```python
from build123d import *

# Parameters (mm, degrees)
F0_W      = 152.4
F0_H      = 152.4
F0_W_2    = 147.32
F0_H_2    = 147.32
F1_DEPTH  = 101.6
F2_W      = 152.4
F2_H      = 152.4
F3_DEPTH  = 2.54
F4_W      = 27.94
F4_H      = 18.1844604351
F4_H_2    = 17.9737907264
F5_DEPTH  = 25.4
F7_DEPTH  = 101.6
F8_W      = 25.4
F8_H      = 5.08
F9_DEPTH  = 101.6
F10_W     = 25.4
F10_H     = 5.08
F11_DEPTH = 101.6
F12_W     = 5.08
F12_H     = 5.08
F13_DEPTH = 101.6
F14_W     = 38.1
F14_H     = 5.08
F15_DEPTH = 101.6
F16_W     = 5.08
F16_H     = 38.4063468442
F16_H_2   = 5.08
F17_DEPTH = 101.6
F18_W     = 25.4
F18_H     = 104.14
F19_DEPTH = 25.4
F20_R     = 5.07999
F21_W     = 5.08
F21_H     = 5.08
F21_W_2   = 38.1
F21_H_2   = 22.86
F22_DEPTH = 101.6
F23_R     = 1.016
F24_DEPTH = 15.24


# Not quite as in the source:
# - a fillet or chamfer is up to 0.001 mm smaller than in the source, because OpenCascade refuses the exact size


with BuildPart() as f1:
    # F0 (on Top) → F1 (new body)
    with BuildSketch(Plane.XY):
        with Locations((-4.47035e-05, 5.21541e-05)):
            Rectangle(F0_W, F0_H)
        with Locations((-4.47035e-05, 5.21541e-05)):
            Rectangle(F0_W_2, F0_H_2, mode=Mode.SUBTRACT)
    extrude(amount=F1_DEPTH)

    # F2 (on face) → F3 (join)
    with BuildSketch(Plane(origin=(0, 0, 0), x_dir=(1, 0, 0), z_dir=(0, 0, -1))):
        with Locations((-4.47035e-05, -5.21541e-05)):
            Rectangle(F2_W, F2_H)
    extrude(amount=F3_DEPTH)

    # F4 (on face) → F5 (cut)
    with BuildSketch(Plane.XZ.offset(76.1999478459)):
        with Locations((44.4499552965, 25.6276302175)):
            Rectangle(F4_W, F4_H)
        with Locations((-44.4500447035, 25.5222953632)):
            Rectangle(F4_W, F4_H_2)
    extrude(amount=-F5_DEPTH, mode=Mode.SUBTRACT)

    # F6 (on face) → F7 (join)
    with BuildSketch(Plane.XY):
        Polygon((-17.7800447035, 58.4200521541), (-17.7800447035, -50.7999478459), (-12.7000447035, -50.7999478459), (-12.7000447035, 53.3400521541), (12.6999552965, 53.3400521541), (12.6999552965, -50.7999478459), (17.7799552965, -50.7999478459), (17.7799552965, 44.5264838636), (17.7799552965, 58.4200521541), align=None)
    extrude(amount=F7_DEPTH)

    # F8 (on face) → F9 (join)
    with BuildSketch(Plane.XY):
        with Locations((-4.47035e-05, -48.2599478459)):
            Rectangle(F8_W, F8_H)
    extrude(amount=F9_DEPTH)

    # F10 (on face) → F11 (cut)
    with BuildSketch(Plane.XY.offset(101.6)):
        with Locations((-4.47035e-05, 55.8800521541)):
            Rectangle(F10_W, F10_H)
    extrude(amount=-F11_DEPTH, mode=Mode.SUBTRACT)

    # F12 (on face) → F13 (join)
    with BuildSketch(Plane.XY):
        with Locations((-20.3200447035, 14.9337053099)):
            Rectangle(F12_W, F12_H)
    extrude(amount=F13_DEPTH)

    # F14 (on face) → F15 (join)
    with BuildSketch(Plane.XY):
        with Locations((-54.6100447035, 14.9337053099)):
            Rectangle(F14_W, F14_H)
    extrude(amount=F15_DEPTH)

    # F16 (on face) → F17 (join)
    with BuildSketch(Plane.XY):
        with Locations((-43.1800447035, 36.676878732)):
            Rectangle(F16_W, F16_H)
        with Locations((-43.1800447035, 71.1200521541)):
            Rectangle(F16_W, F16_H_2)
        with Locations((43.1799552965, 71.1200521541)):
            Rectangle(F16_W, F16_H_2)
        with Locations((43.1799552965, 36.676878732)):
            Rectangle(F16_W, F16_H)
    extrude(amount=F17_DEPTH)

    # F18 (on face) → F19 (cut)
    with BuildSketch(Plane.XY):
        with Locations((-4.47035e-05, 6.3500521541)):
            Rectangle(F18_W, F18_H)
    extrude(amount=-F19_DEPTH, mode=Mode.SUBTRACT)

    # F20 (radius 5.08 in the source; OpenCascade refuses exactly that, so slightly less here)
    f20_edges = [f1.edges().sort_by_distance(p)[0] for p in [
        (-17.780045, 58.420052, 50.8),
        (17.779955, 58.420052, 50.8),
    ]]
    fillet(f20_edges, radius=F20_R)

    # F21 (on face) → F22 (join)
    with BuildSketch(Plane.XY):
        with Locations((20.3199552965, 14.9337053099)):
            Rectangle(F21_W, F21_H)
        with Locations((54.6099552965, 14.9337053099)):
            Rectangle(F21_W_2, F21_H)
        with Locations((-15.2400447035, -62.2299478459)):
            Rectangle(F21_W, F21_H_2)
        with Locations((15.2399552965, -71.1199478459)):
            Rectangle(F21_W, F21_H)
    extrude(amount=F22_DEPTH)

    # F23 (on face) → F24 (cut)
    with BuildSketch(Plane(origin=(0, 0, -2.54), x_dir=(1, 0, 0), z_dir=(0, 0, -1))):
        with Locations((-74.9300447035, 74.9299478459)):
            Circle(F23_R)
        with Locations((74.9299552965, 74.9299478459)):
            Circle(F23_R)
        with Locations((-74.9300447035, -74.9300521541)):
            Circle(F23_R)
        with Locations((74.9299552965, -74.9300521541)):
            Circle(F23_R)
    extrude(amount=-F24_DEPTH, mode=Mode.SUBTRACT)


solid = f1.part
```
Build history of the part. All positions in model axes, mm. A direction names the side the tool comes from. Round coordinates to 2 decimals unless told otherwise and drop trailing zeros. Write each loop counter-clockwise with the first axis right and the second up, starting at its lowest first coordinate (ties: lowest second). Pieces come first, ordered by that corner, then holes.
1) Band-saw the part on A-A, the plane x = -9. List the corners of the cut face in (y, z), and give its area (3 significant figures).
2) Band-saw the part on B-B, the plane y = 41.5. List the corners of the cut face in (x, z), and give its area (3 significant figures).
3) Drill centre lines: probe 1 along X at (y, z) = (70, 89.5); probe 2 along Y at (x, z) = (7, 63.5); probe 3 along X at (y, z) = (31, 22). Where is each one in solid material? Low to high.
4) Mould opens along Y. For faces 3 (the flat face through (20, 12.394, 50)), 4 (the flat face through (-76.2, 1, 50)) say: +Y half, -Y half, draft (parallel to the pull), parting line (faces both ways), or undercut.
5) Pin check, flat tips, straight feed: pin 1 (0.6 mm diameter, centred on x = -74.5, y = -74.5, fed in from -Z); pin 2 (4 mm diameter, centred on x = 40.5, y = -23, fed in from +Z). Stop position of each tip, or through.
6) Band-saw the part on D-D, the plane x = 53. List the corners of the cut face in (y, z), and give its area (3 significant figures).
7) 3-axis set-ups, long thin cutter, end or side, ignore diameter. For faces 1 (the flat face through (73.66, 45, 50)), 2 (the flat face through (-12.7, 6, 50)): which of +Z, -Z, +X, -X, +Y, -Y reach the whole face in a straight line?
8) Band-saw the part on C-C, the plane y = -59. List the corners of the cut face in (x, z).
Ans:
1. outline: (-76.2, -2.54) - (-45.72, -2.54) - (-45.72, 101.6) - (-50.8, 101.6) - (-50.8, 0) - (-73.66, 0) - (-73.66, 101.6) - (-76.2, 101.6) - close; (58.42, -2.54) - (76.2, -2.54) - (76.2, 101.6) - (73.66, 101.6) - (73.66, 0) - (58.42, 0) - close
1. area: 1,150 mm2
2. outline: (-76.2, -2.54) - (-12.7, -2.54) - (-12.7, 101.6) - (-17.78, 101.6) - (-17.78, 0) - (-40.64, 0) - (-40.64, 101.6) - (-45.72, 101.6) - (-45.72, 0) - (-73.66, 0) - (-73.66, 101.6) - (-76.2, 101.6) - close; (12.7, -2.54) - (76.2, -2.54) - (76.2, 101.6) - (73.66, 101.6) - (73.66, 0) - (45.72, 0) - (45.72, 101.6) - (40.64, 101.6) - (40.64, 0) - (17.78, 0) - (17.78, 101.6) - (12.7, 101.6) - close
2. area: 2,900 mm2
3. probe 1: x = -76.2 to -73.66, -45.72 to -40.64, 40.64 to 45.72, 73.66 to 76.2
3. probe 2: y = -76.2 to -73.66, -50.8 to -45.72, 73.66 to 76.2
3. probe 3: x = -76.2 to -73.66, -45.72 to -40.64, -17.78 to -12.7, 12.7 to 17.78, 40.64 to 45.72, 73.66 to 76.2
4. face 3: undercut
4. face 4: draft
5. pin 1: stops at z = 12.7
5. pin 2: stops at z = 0
6. outline: (-76.2, -2.54) - (76.2, -2.54) - (76.2, 101.6) - (73.66, 101.6) - (73.66, 0) - (17.47, 0) - (17.47, 101.6) - (12.39, 101.6) - (12.39, 0) - (-73.66, 0) - (-73.66, 16.54) - (-76.2, 16.54) - close; (-76.2, 34.72) - (-73.66, 34.72) - (-73.66, 101.6) - (-76.2, 101.6) - close
6. area: 1,370 mm2
7. face 1: +Z
7. face 2: +Z, -Z
8. outline: (-76.2, -2.54) - (76.2, -2.54) - (76.2, 101.6) - (73.66, 101.6) - (73.66, 0) - (-12.7, 0) - (-12.7, 101.6) - (-17.78, 101.6) - (-17.78, 0) - (-73.66, 0) - (-73.66, 101.6) - (-76.2, 101.6) - close
